Verification items for the finished model (mm, model axes). A direction names the side the tool comes from. Give positions to 0.01 mm unless a question says otherwise; leave off trailing zeros. Order: outer loops, then holes, each group sorted by start corner. A loop starts at its lowest first (then second) coordinate and runs counter-clockwise, first axis right, second up.
(1) Sectioned sample at A-A on y = 17.5. Record the cut outline in (x, z), plus the area to 3 significant figures.
(2) Gauge pin test, flat ends, axial feed: pin 1 (6 mm diameter, centred on y = 12, z = -10.5, fed in from +X); pin 2 (6 mm diameter, centred on x = 12.5, y = 25, fed in from +Z); pin 3 (3 mm diameter, centred on y = 15.5, z = 8, fed in from +X); pin 4 (17 mm diameter, centred on x = -25.5, z = -66.5, fed in from -Y). Record the tip position at first contact, or that the pin passes through.
(3) Access from +Z, -Z, +X, -X, +Y, -Y to the whole of each face (thin tool, end or side, straight path). Record for faces 4 (the face through (44.59, 20.25, -49.77)), 5 (the face through (-42, 20, -25.608)), 6 (the face through (9.586, 33.666, -74.119)), 7 (the face through (-7, 0, -39)), 8 (the face through (-42, 18, 9.394)).
(4) Sectioned sample at C-C on y = 29. Record the cut outline in (x, z), plus the area to 3 significant figures.
(5) Mould release check, pull along X, two halves, no side actions. Record for faces 1 (the face through (-12, 31, -55)), 2 (the face through (-42, 27.5, -19)), 3 (the face through (-41.559, 20, 7)): pulls with the +X half, pulls with the -X half, needs draft (parallel to the pull), parting line crosses it, or undercut.
(6) Sectioned sample at D-D on x = 37.5. Record the cut outline in (y, z), plus the area to 3 significant figures.
(7) Sectioned sample at B-B on z = -16.5. Record the cut outline in (x, y).
(8) Scan lines: L1, parallel to Y at x = 10, z = -23.5; L2, parallel to Y at x = 3.5, z = -70.5; L3, parallel to X at y = 13, z = -51. Record each from-to range of solid material in increasing order.
```python
from build123d import *

# Parameters (mm, degrees)
BOSS_EXTRUDE1_DEPTH = 40
SHELL1_T            = -3
BOSS_EXTRUDE2_DEPTH = 4
BOSS_EXTRUDE3_DEPTH = 4
BOSS_EXTRUDE4_DEPTH = 1.8
BOSS_EXTRUDE5_DEPTH = 1.8
SKETCH10_R          = 1.6
CUT_EXTRUDE6_DEPTH  = 107.30423742
SKETCH11_W          = 12.8
SKETCH11_H          = 15
CUT_EXTRUDE7_DEPTH  = 3
BOSS_EXTRUDE7_START = 10
SKETCH12_W          = 69.967359313
SKETCH12_H          = 34
SKETCH12_R          = 1.6
BOSS_EXTRUDE7_DEPTH = 10
SKETCH13_R          = 3.1
CUT_EXTRUDE9_DEPTH  = 10
SKETCH14_W          = 69.967359313
SKETCH14_H          = 22
CUT_EXTRUDE10_DEPTH = 10


with BuildPart() as part:
    # Sketch1 → Boss-Extrude1 (new body)
    with BuildSketch(Plane(origin=(0, 0, 0), x_dir=(1, 0, 0), z_dir=(0, 1, 0))):
        Polygon((-43.359374855, -5.394325428), (-43.359374855, 35.316352691), (9.115019377, 87.790746923), (44.470358437, 52.435407864), (-13.359374855, -5.394325428), align=None)
    extrude(amount=BOSS_EXTRUDE1_DEPTH)

    # Shell1
    shell1_openings = [part.faces().sort_by_distance(p)[0] for p in [
        (15.555491791, 20, -23.520541218),
        (-28.359374855, 20, 5.394325428),
    ]]
    offset(amount=SHELL1_T, openings=shell1_openings, kind=Kind.INTERSECTION)

    # Sketch6 → Boss-Extrude2 (add)
    with BuildSketch(Plane(origin=(-3.982524714, 0, -3.982524714), x_dir=(0.7071067811865489, 0, -0.7071067811865462), z_dir=(0.7071067811865462, 0, 0.7071067811865489))):
        Polygon((-13.260868642, 38.2), (66.722724487, 38.2), (66.722724487, 1.8), (-13.260868642, 1.8), (-13.260868642, 0), (68.522724487, 0), (68.522724487, 40), (-13.260868642, 40), align=None)
    extrude(amount=BOSS_EXTRUDE2_DEPTH)

    # Sketch7 → Boss-Extrude3 (add)
    with BuildSketch(Plane.XY.offset(5.394325428)):
        Polygon((-13.359374855, 1.8), (-41.559374855, 1.8), (-41.559374855, 38.2), (-13.359374855, 38.2), (-13.359374855, 40), (-43.359374855, 40), (-43.359374855, 0), (-13.359374855, 0), align=None)
    extrude(amount=BOSS_EXTRUDE3_DEPTH)

    # Sketch8 → Boss-Extrude4 (add)
    with BuildSketch(Plane.XZ):
        Polygon((-13.359374855, 9.394325428), (-11.702520605, 9.394325428), (-10.53094773, 8.222752552), (-13.359374855, 5.394325428), align=None)
    extrude(amount=-BOSS_EXTRUDE4_DEPTH)

    # Sketch9 → Boss-Extrude5 (add)
    with BuildSketch(Plane(origin=(0, 40, 0), x_dir=(1, 0, 0), z_dir=(0, 1, 0))):
        Polygon((-13.359374855, -5.394325428), (-10.53094773, -8.222752552), (-11.553745116, -9.245549939), (-13.359374855, -9.394325428), align=None)
    extrude(amount=-BOSS_EXTRUDE5_DEPTH)

    # Sketch10 → Cut-Extrude6 (cut, through all)
    with BuildSketch(Plane(origin=(-37.216543429, 0, -37.216543429), x_dir=(0.7071067811865488, 0, -0.7071067811865464), z_dir=(0.7071067811865464, 0, 0.7071067811865488))):
        with Locations((60.522724487, 35)):
            Circle(SKETCH10_R)
        with Locations((60.522724487, 5)):
            Circle(SKETCH10_R)
        with Locations((0.522724487, 35)):
            Circle(SKETCH10_R)
        with Locations((0.522724487, 5)):
            Circle(SKETCH10_R)
    extrude(amount=-CUT_EXTRUDE6_DEPTH, mode=Mode.SUBTRACT)

    # Sketch11 → Cut-Extrude7 (cut)
    with BuildSketch(Plane(origin=(-40.359374855, 0, 0), x_dir=(0, 0, -1), z_dir=(1, 0, 0))):
        with Locations((19.207640819, 20)):
            Rectangle(SKETCH11_W, SKETCH11_H)
    extrude(amount=-CUT_EXTRUDE7_DEPTH, mode=Mode.SUBTRACT)

    # Sketch12 → Boss-Extrude7 (add)
    with BuildSketch(Plane(origin=(-37.216543429, 0, -37.216543429), x_dir=(0.7071067811865488, 0, -0.7071067811865464), z_dir=(0.7071067811865464, 0, 0.7071067811865488)).offset(BOSS_EXTRUDE7_START)):
        with Locations((30.539044831, 20)):
            Rectangle(SKETCH12_W, SKETCH12_H)
        with Locations((0.522724487, 35)):
            Circle(SKETCH12_R, mode=Mode.SUBTRACT)
        with Locations((60.522724487, 35)):
            Circle(SKETCH12_R, mode=Mode.SUBTRACT)
        with Locations((60.522724487, 5)):
            Circle(SKETCH12_R, mode=Mode.SUBTRACT)
        with Locations((0.522724487, 5)):
            Circle(SKETCH12_R, mode=Mode.SUBTRACT)
    extrude(amount=-BOSS_EXTRUDE7_DEPTH)

    # Sketch13 → Cut-Extrude9 (cut)
    with BuildSketch(Plane(origin=(-39.337863773, 0, -39.337863773), x_dir=(-0.7071067811865488, 0, 0.7071067811865464), z_dir=(-0.7071067811865464, 0, -0.7071067811865488))):
        with Locations((-0.522724487, 35)):
            Circle(SKETCH13_R)
        with Locations((-0.522724487, 5)):
            Circle(SKETCH13_R)
        with Locations((-60.522724487, 5)):
            Circle(SKETCH13_R)
        with Locations((-60.522724487, 35)):
            Circle(SKETCH13_R)
    extrude(amount=-CUT_EXTRUDE9_DEPTH, mode=Mode.SUBTRACT)

    # Sketch14 → Cut-Extrude10 (cut)
    with BuildSketch(Plane(origin=(-30.145475617, 0, -30.145475617), x_dir=(0.7071067811865488, 0, -0.7071067811865462), z_dir=(0.7071067811865462, 0, 0.7071067811865488))):
        with Locations((30.539044831, 20)):
            Rectangle(SKETCH14_W, SKETCH14_H)
    extrude(amount=-CUT_EXTRUDE10_DEPTH, mode=Mode.SUBTRACT)


solid = part.part
```
Ans:
1. outline: (-43.36, -35.32) - (9.12, -87.79) - (47.3, -49.61) - (46.03, -48.33) - (43.2, -51.16) - (42.35, -50.31) - (9.12, -83.55) - (-40.36, -34.07) - (-40.36, -25.61) - (-43.36, -25.61) - close; (-43.36, -12.81) - (-40.36, -12.81) - (-40.36, 5.39) - (-41.56, 5.39) - (-41.56, 9.39) - (-43.36, 9.39) - close
1. area: 458 mm2
2. pin 1: stops at x = -40.36
2. pin 2: stops at z = -77.16
2. pin 3: stops at x = -41.56
2. pin 4: passes through
3. face 4: +Z
3. face 5: +X, -X
3. face 6: none
3. face 7: +Z, -Z, +X, -X, -Y
3. face 8: +Z, +X, -X, +Y, -Y
4. outline: (-43.36, -35.32) - (9.12, -87.79) - (47.3, -49.61) - (46.03, -48.33) - (43.2, -51.16) - (42.35, -50.31) - (9.12, -83.55) - (-40.36, -34.07) - (-40.36, 5.39) - (-41.56, 5.39) - (-41.56, 9.39) - (-43.36, 9.39) - close
4. area: 496 mm2
5. face 1: undercut
5. face 2: needs draft
5. face 3: pulls with the +X half
6. outline: (0, -59.41) - (40, -59.41) - (40, -39.81) - (38.2, -39.81) - (38.2, -45.47) - (37, -45.47) - (37, -55.16) - (3, -55.16) - (3, -45.47) - (1.8, -45.47) - (1.8, -39.81) - (0, -39.81) - close
6. area: 248 mm2
7. outline: (-43.36, 0) - (14.19, 0) - (14.19, 1.8) - (8.53, 1.8) - (8.53, 3) - (-40.36, 3) - (-40.36, 12.5) - (-43.36, 12.5) - close; (-43.36, 27.5) - (-40.36, 27.5) - (-40.36, 37) - (8.53, 37) - (8.53, 38.2) - (14.19, 38.2) - (14.19, 40) - (-43.36, 40) - close
8. L1: y = 0 to 3, 37 to 40
8. L2: y = 0 to 9, 31 to 40
8. L3: x = -27.68 to -23.43, 41.66 to 43.03, 43.36 to 45.91
